The listing builds one solid part. Answer for the finished solid, in the listing's coordinates (mm). Face numbers are marked on the shaded views. A direction names the side the tool comes from. Round coordinates to 2 decimals unless told otherwise and drop trailing zeros. Loops run counter-clockwise (first coordinate to the right, second up) from the corner with the lowest first, then second, coordinate; pieces in that order, holes last. Notation, with made-up numbers: (-14, 9.5) - (21, 9.5) arc R23 ccw to (21, 28.5) - close; hole circle Ø11 at (-0.5, -8.75). An arc over 180 degrees is marked (long way). One line per item, written item: value.
```python
from build123d import *

# Parameters (mm, degrees)
F2_R     = 19.00963
F3_DEPTH = 50.9


with BuildPart() as f1:
    # F0 (on Front) → F1 (revolve)
    with BuildSketch(Plane.XZ):
        Polygon((-48, 4), (-48, 3.5), (0, 3.5), (0, 4), (-4.333333, 5), (-4.333333, 4), (-8.666667, 5), (-8.666667, 4), (-13, 5), (-17, 5), (-17, 9), (-21, 9), (-21, 5), (-24.175, 5), (-24.175, 5.5), (-24.675, 5.5), (-24.675, 9), (-28.675, 9), (-28.675, 5.5), (-33.675, 5.5), (-33.675, 5), (-38.45, 4), (-38.45, 5), (-43.225, 4), (-43.225, 5), align=None)
    revolve(axis=Axis((-24, 0, 0), (-1, 0, 0)))

    # F2 (on Right) → F3 (cut)
    with BuildSketch(Plane.YZ):
        Circle(F2_R)
        Polygon((0.801815, 9.20274), (8.370714, 3.906978), (7.568899, -5.295762), (-0.801815, -9.20274), (-8.370714, -3.906978), (-7.568899, 5.295762), align=None, mode=Mode.SUBTRACT)
    extrude(amount=-F3_DEPTH, mode=Mode.SUBTRACT)


solid = f1.part
```
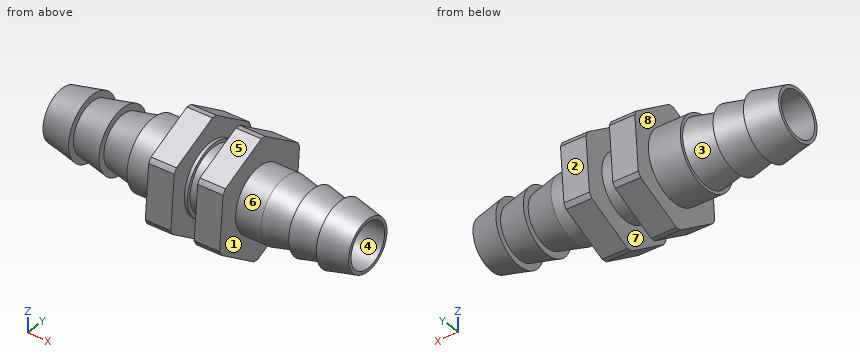
1) A cutting plane is placed at C-C on z = -6. Give the vertices of the cut face in (x, y) (3 decimals), and give its area (3 significant figures).
Final values:
outline: (-28.675, -5.379) - (-24.675, -5.379) - (-24.675, 6.06) - (-28.675, 6.06) - close; (-21, -5.379) - (-17, -5.379) - (-17, 6.06) - (-21, 6.06) - close
area: 91.5 mm2
2) For the marked faces 4, 5, 6, 7 and 8, determine the directions among +Z, -Z, +X, -X, +Y, -Y from which every point of the face is accessible in a straight line to the end or side of a thin tool.
Final values:
face 4: +X, -X
face 5: +Z, +X, -X, -Y
face 6: +X
face 7: none
face 8: -X
3) A cutting plane is placed at A-A on y = 6. Give the vertices of the cut face in (x, z) (3 decimals).
Final values:
outline: (-28.675, -6.028) - (-24.675, -6.028) - (-24.675, 5.566) - (-28.675, 5.566) - close; (-21, -6.028) - (-17, -6.028) - (-17, 5.566) - (-21, 5.566) - close
4) A cutting plane is placed at D-D on x = -38. Give the vertices of the cut face in (y, z), and give its area (3 significant figures).
Final values:
outline: circle Ø8.19 at (0, 0); hole circle Ø7 at (0, 0)
area: 14.2 mm2
5) Each of these flat-tipped pins is pushed along its axis until it touches: pin 1 Ø8 at (x, y) = (-9, -2.5) entering from +Z; pin 2 Ø8 at (x, y) = (-42, 4) entering from -Z; pin 3 Ø1.5 at (x, z) = (-7.5, 1.5) entering from -Y. Where does it stop, or does it pass through?
Final values:
pin 1: z = 5
pin 2: z = -5
pin 3: y = -4.76
6) Consider L1, parallel to X at y = -6.5, z = 2.25 (3 decimals); L2, parallel to Y at x = -23.5, z = 0; L3, parallel to Y at x = -31.5, z = 0. Determine where each line is inside the solid, lowest interval first.
Final values:
L1: -28.675 to -24.675, -21 to -17
L2: -5 to -3.5, 3.5 to 5
L3: -5.5 to -3.5, 3.5 to 5.5
7) A cutting plane is placed at B-B on x = -18.5. Give the vertices of the cut face in (y, z), and give its area (3 significant figures).
Final values:
outline: (-8.33, -3.41) arc R9 ccw to (-7.96, -4.19) - (-1.21, -8.92) arc R9 ccw to (-0.35, -8.99) - (7.12, -5.51) arc R9 ccw to (7.61, -4.8) - (8.33, 3.41) arc R9 ccw to (7.96, 4.19) - (1.21, 8.92) arc R9 ccw to (0.35, 8.99) - (-7.12, 5.51) arc R9 ccw to (-7.61, 4.8) - close; hole circle Ø7 at (0, 0)
area: 183 mm2
8) For a pull along X with two mould halves and no side action, classify the marked faces 1, 2 and 3 as released by +X, released by -X, zero draft, split by the parting line, or undercut.
Final values:
face 1: released by +X
face 2: zero draft
face 3: undercut
